from build123d import *

# Parameters (mm, degrees)
SKETCH1_R               = 13
SKETCH1_R_2             = 3
BOSS_EXTRUDE1_DEPTH     = 25
SKETCH2_W               = 15.5
SKETCH2_H               = 13.6
CUT_EXTRUDE1_DEPTH      = 6.85
CUT_EXTRUDE2_REACH      = 33.032
CUT_EXTRUDE2_END_RADIUS = 13


with BuildPart() as part:
    # Sketch1 → Boss-Extrude1 (new body)
    with BuildSketch(Plane.XY):
        Circle(SKETCH1_R)
        Circle(SKETCH1_R_2, mode=Mode.SUBTRACT)
    extrude(amount=BOSS_EXTRUDE1_DEPTH)

    # Sketch2 → Cut-Extrude1 (cut, symmetric)
    with BuildSketch(Plane(origin=(0, 0, 0), x_dir=(1, 0, 0), z_dir=(0, 1, 0))):
        with Locations((0, -18.2)):
            Rectangle(SKETCH2_W, SKETCH2_H)
    extrude(amount=CUT_EXTRUDE1_DEPTH, both=True, mode=Mode.SUBTRACT)

    # Cut-Extrude2: up to this cylinder (the profile starts inside it)
    cut_extrude2_end = Plane(origin=(0, 0, 19.701869), z_dir=(0, 0, -1)) * Cylinder(CUT_EXTRUDE2_END_RADIUS, 93.064, mode=Mode.PRIVATE)
    # Sketch3 → Cut-Extrude2 (cut, up to the surface)
    with BuildSketch(Plane(origin=(0, 0, 0), x_dir=(1, 0, 0), z_dir=(0, 1, 0)), mode=Mode.PRIVATE) as cut_extrude2_sk1:
        with BuildLine():
            Line((-6.95, -18.2), (-6.95, -25))
            Line((-6.95, -25), (2.45, -25))
            Line((2.45, -25), (2.45, -18.2))
            ThreePointArc((2.45, -18.2), (-2.25, -13.5), (-6.95, -18.2))
        make_face()
    cut_extrude2_tool1 = extrude(cut_extrude2_sk1.sketch, amount=-CUT_EXTRUDE2_REACH, mode=Mode.PRIVATE) & cut_extrude2_end
    add(cut_extrude2_tool1.solids().sort_by_distance((-2.25, 0, 19.701869))[0], mode=Mode.SUBTRACT)


solid = part.part
Model file for the job. Use its own axes, mm. A direction names the side the tool comes from. Give positions to 0.01 mm unless a question says otherwise; leave off trailing zeros. Loops run counter-clockwise (first coordinate to the right, second up) from the corner with the lowest first, then second, coordinate; pieces in that order, holes last. Notation, with made-up numbers: (-15.75, 78.5) - (-0.75, 78.5) arc R12 cw to (-0.75, 87.5) - close; hole circle Ø8 at (48.25, 25). An arc over 180 degrees is marked (long way). Use one line per item in the form item = value.
(1) Cut at C-C (y = -5). Give the cut face in (x, z), then the cut area to 3 significant figures.
Determined:
outline = (-12, 0) - (12, 0) - (12, 25) - (7.75, 25) - (7.75, 11.4) - (-7.75, 11.4) - (-7.75, 25) - (-12, 25) - close
area = 389 mm^2
(2) Pull direction X, two halves, no side cores. Call faces 4 (the face through (-3, 0, 6)), 5 (the face through (0, 9, 25)), 6 (the face through (2.45, -10, 22)), 7 (the face through (-1.69, 12.89, 12.32)): pulls with the +X half, pulls with the -X half, needs draft (parallel to the pull), parting line crosses it, or undercut.
Determined:
face_4 = undercut
face_5 = needs draft
face_6 = undercut
face_7 = parting line crosses it
(3) Cut at D-D (z = 22.75). Give the cut face in (x, y).
Determined:
outline = (-7.75, -6.85) - (-7.75, 6.85) - (7.75, 6.85) - (7.75, -6.85) - (2.45, -6.85) - (2.45, -12.77) arc R13 ccw (long way) to (-6.95, -10.99) - (-6.95, -6.85) - close
(4) Cut at B-B (x = -2.25). Give the cut face in (y, z), then the cut area to 3 significant figures.
Determined:
outline = (-12.8, 0) - (-1.98, 0) - (-1.98, 11.4) - (-6.85, 11.4) - (-6.85, 13.5) - (-12.8, 13.5) - close; (1.98, 0) - (12.8, 0) - (12.8, 25) - (6.85, 25) - (6.85, 11.4) - (1.98, 11.4) - close
area = 340 mm^2
(5) 3-axis set-ups, long thin cutter, end or side, ignore diameter. For faces 1 (the face through (3, -3, 0)), 2 (the face through (3.3, 0.1, 11.4)), 3 (the face through (-6.95, -9, 22)): which of +Z, -Z, +X, -X, +Y, -Y reach the whole face in a straight line?
Determined:
face_1 = -Z, +X, -X, +Y, -Y
face_2 = +Z
face_3 = +Z, -Y
(6) Drill centre lines: L1, parallel to X at y = 0, z = 5.75; L2, parallel to X at y = 1.25, z = 6. Where is each one in solid material? Low to high.
Determined:
L1 = -13 to -3, 3 to 13
L2 = -12.94 to -2.73, 2.73 to 12.94
(7) Cut at A-A (y = 0). Give the cut face in (x, z), then the cut area to 3 significant figures.
Determined:
outline = (-13, 0) - (-3, 0) - (-3, 11.4) - (-7.75, 11.4) - (-7.75, 25) - (-13, 25) - close; (3, 0) - (13, 0) - (13, 25) - (7.75, 25) - (7.75, 11.4) - (3, 11.4) - close
area = 371 mm^2
(8) Drop flat-ended pins along their axis: P1, Ø1.5, axis at x = 1.5, y = 0, coming from the -Z side; P2, Ø1, axis at x = 4, z = 5.5, coming from the +Y side; P3, Ø5, axis at x = 4, z = 11.5, coming from the -Y side; P4, Ø4, axis at y = 8, z = 7, coming from the -X side. Give the stop position or say it passes through.
Determined:
P1 = through
P2 = 12.52
P3 = -12.91
P4 = -11.53
